Here's how the part is built. I have some questions about the finished solid (model axes, mm). A direction names the side the tool comes from. Coordinates: 2 decimals unless noted, no trailing zeros. Write each loop counter-clockwise with the first axis right and the second up, starting at its lowest first coordinate (ties: lowest second). Pieces come first, ordered by that corner, then holes.
Item 1: If we mould it in two halves opening along Z, with no side actions, what happens to faces 1 (the face through (0, 9, -8)), 2 (the face through (4.585, 11.007, 13.864)), 3 (the face through (-7.5, 9, 1))? For each: pulls with the +Z half, pulls with the -Z half, needs draft (parallel to the pull), parting line crosses it, or undercut.
Item 2: I want a section at A-A (y = 4.5). Please give me the cut outline in (x, z), and give its area (3 significant figures).
Item 3: Please list where these lines run through material, in increasing order: line 1 (X direction, y = 11.25, z = 15.5); line 2 (Z direction, x = 4.8, y = 10.8); line 3 (Z direction, x = 4, y = 5).
Item 4: I want a section at B-B (z = 0). Please give me the cut outline in (x, y).
Item 5: I want a section at C-C (x = 0.25). Please give me the cut outline in (y, z).
Item 6: I'm going to push flat-ended pins straight in: P1, Ø4, axis at y = 8, z = 17.5, coming from the +X side; P2, Ø6.5, axis at y = 4.5, z = 15.5, coming from the -X side; P3, Ø3.5, axis at x = -4, z = 16, coming from the +Y side; P4, Ø2, axis at x = -1, y = 6, coming from the +Z side. Where does each tip first touch, or does it pass through?
Item 7: I want a section at D-D (y = 15.25). Please give me the cut outline in (x, z), and give its area (3 significant figures).
Item 8: For faces 4 (the face through (-5.015, 11.007, 13.864)), 5 (the face through (7.5, 9, 2)), 6 (the face through (2, 11.5, 16)), 7 (the face through (0, 5, 11.5)), which set-ups out of +Z, -Z, +X, -X, +Y, -Y let a thin tool reach every point of the face, with its end or its side?
Autodesk Inventor part; units mm, degrees
ref_plane "YZ Plane" through (0, 0, 0) normal (1, 0, 0) x (0, 1, 0)
ref_plane "XZ Plane" through (0, 0, 0) normal (0, 1, 0) x (-1, 0, 0)
ref_plane "XY Plane" through (0, 0, 0) normal (0, 0, 1) x (1, 0, 0)
sketch "Sketch1" plane through (0, 0, 0) normal (0, 1, 0) x (-1, 0, 0)
  line L0 (8.5, 21.5) -> (-8.5, 21.5)
  line L1 (-8.5, 21.5) -> (-8.5, -21.5)
  line L2 (-8.5, -21.5) -> (8.5, -21.5)
  line L3 (8.5, -21.5) -> (8.5, 21.5)
  line L4 (-8.5, 21.5) -> (8.5, -21.5) construction
  point P0 (0, 0)
  point P1 (0, 0)
  dimension "d0" = 43
  dimension "d1" = 17
extrude "Extrusion1" add sketch "Sketch1" along normal blind 1.5
sketch "Sketch2" plane through (0, 1.5, 0) normal (0, 1, 0) x (1, 0, 0)
  line L0 (-7.5, -11) -> (7.5, -11)
  line L1 (7.5, -11) -> (7.5, 8)
  line L2 (7.5, 8) -> (-7.5, 8)
  line L3 (-7.5, 8) -> (-7.5, -11)
  line L4 (-8.5, -21.5) -> (8.5, -21.5)
  point P0 (0, 0)
  dimension "d4" = 19
  dimension "d5" = 15
  dimension "d6" = 7.5
  dimension "d8" = 10.5
extrude "Extrusion2" add sketch "Sketch2" along normal blind 15
sketch "Sketch3" plane through (0, 1.5, 0) normal (0, 1, 0) x (1, 0, 0)
  line L0 (7.5, -11.5) -> (-7.5, -11.5)
  line L1 (-7.5, -11.5) -> (-7.5, -19.5)
  line L2 (-7.5, -19.5) -> (7.5, -19.5)
  line L3 (7.5, -19.5) -> (7.5, -11.5)
  line L4 (-7.5, -11) -> (7.5, -11)
  point P0 (0, 0)
  dimension "d11" = 15
  dimension "d12" = 8
  dimension "d13" = 0.5
  dimension "d14" = 7.5
extrude "Extrusion3" add sketch "Sketch3" along normal blind 10
chamfer "Chamfer1" distance 1 distance2 3.5 1 edges at (0, 11.5, 19.5) measured on face at (2.5, 11.5, 16.8333)
chamfer "Chamfer2" distance 1 distance2 3.5 1 edges at (0, 11.5, 11.5) measured on face at (2.5, 11.5, 16.1667)
sketch "Sketch4" plane through (0, 11.5, 0) normal (0, 1, 0) x (1, 0, 0)
  circle A0 centre (-4.8, -15.5) radius 1.65
  line L0 (-7.5, -12.5) -> (-7.5, -18.5)
  line L1 (-3.2324, -14.8041) -> (3.2927, -14.8041) construction
  circle A1 centre (0, -15.5) radius 1.65
  circle A2 centre (4.8, -15.5) radius 1.65
  point P0 (0, 0)
  dimension "d23" = 3.3
  dimension "d24" = 2.7
  dimension "d27" = 4.8
  dimension "d32" = 6
  dimension "d33" = 3
extrude "Extrusion4" cut sketch "Sketch4" against normal blind 1
equation "\"d33\" = 0.5 * d32"
properties part number "Relay w Breakout Board"
Answer:
1. face 1: pulls with the -Z half
1. face 2: undercut
1. face 3: needs draft
2. outline: (-7.5, -8) - (7.5, -8) - (7.5, 11) - (-7.5, 11) - close; (-7.5, 11.5) - (7.5, 11.5) - (7.5, 19.5) - (-7.5, 19.5) - close
2. area: 405 mm2
3. line 1: x = -7.5 to -6.45, -3.15 to -1.65, 1.65 to 3.15, 6.45 to 7.5
3. line 2: z = -8 to 11, 12.3 to 13.85, 17.15 to 18.7
3. line 3: z = -8 to 11, 11.5 to 19.5
4. outline: (-8.5, 0) - (8.5, 0) - (8.5, 1.5) - (7.5, 1.5) - (7.5, 16.5) - (-7.5, 16.5) - (-7.5, 1.5) - (-8.5, 1.5) - close
5. outline: (0, -21.5) - (1.5, -21.5) - (1.5, -8) - (16.5, -8) - (16.5, 11) - (1.5, 11) - (1.5, 11.5) - (8, 11.5) - (11.5, 12.5) - (11.5, 13.87) - (10.5, 13.87) - (10.5, 17.13) - (11.5, 17.13) - (11.5, 18.5) - (8, 19.5) - (1.5, 19.5) - (1.5, 21.5) - (0, 21.5) - close
6. P1: stops at x = 7.5
6. P2: stops at x = -8.5
6. P3: stops at y = 11.5
6. P4: stops at z = 19.5
7. outline: (-7.5, -8) - (7.5, -8) - (7.5, 11) - (-7.5, 11) - close
7. area: 285 mm2
8. face 4: +Y
8. face 5: +Z, -Z, +X, +Y
8. face 6: +Z, +X, -X, +Y
8. face 7: +X, -X, +Y
